Source: CAD feature listing. Evaluate the final solid. Frame: model axes, mm. Give positions to 0.01 mm unless a question says otherwise; leave off trailing zeros. Write each loop counter-clockwise with the first axis right and the second up, starting at its lowest first coordinate (ties: lowest second). Pieces come first, ordered by that corner, then holes. Notation, with made-up numbers: M -7,53 L 22,53 A8 ccw 22,60 Z; hole C -31.5,69 d11. An arc over 180 degrees is marked long. Use CSV: the item, a comma, the result in double quotes. Start each with the question number.
from build123d import *

# Parameters (mm, degrees)
RESSALTO_EXTRUS_O1_DEPTH = 2


with BuildPart() as part:
    # Esboço1 → Ressalto-extrusão1 (new body)
    with BuildSketch(Plane(origin=(0, 0, 0), x_dir=(0, 0, -1), z_dir=(1, 0, 0))):
        with BuildLine():
            Line((0, 0), (-10, 0))
            Line((-10, 0), (-10, 8))
            Line((-10, 8), (-18, 8))
            Line((-18, 8), (-18, 13))
            Line((-18, 13), (-31, 13))
            Line((-31, 13), (-31, 8))
            Line((-31, 8), (-39, 8))
            Line((-39, 8), (-37, 6))
            Line((-37, 6), (-39.121320344, 3.878679656))
            Line((-39.121320344, 3.878679656), (-47.606601718, 12.363961031))
            Line((-47.606601718, 12.363961031), (-60, 12.363961031))
            Line((-60, 12.363961031), (-60.666666667, 10.478342948))
            Line((-60.666666667, 10.478342948), (-63, 11.303300859))
            Line((-63, 11.303300859), (-65.666666667, 3.760828526))
            Line((-65.666666667, 3.760828526), (-63.333333333, 2.935870615))
            Line((-63.333333333, 2.935870615), (-65.303300859, -2.636038969))
            Line((-65.303300859, -2.636038969), (-70, -2.636038969))
            Line((-70, -2.636038969), (-70, 0.363961031))
            Line((-70, 0.363961031), (-77, 0.363961031))
            Line((-77, 0.363961031), (-77, -2.636038969))
            Line((-77, -2.636038969), (-80, -2.636038969))
            Line((-80, -2.636038969), (-78, -9.636038969))
            Line((-78, -9.636038969), (-105.645751311, -9.636038969))
            Line((-105.645751311, -9.636038969), (-106.822875656, -5.813163314))
            Line((-106.822875656, -5.813163314), (-103, -4.636038969))
            Line((-103, -4.636038969), (-104.765686517, 1.098274514))
            Line((-104.765686517, 1.098274514), (-107.645751311, 0.21145666))
            Line((-107.645751311, 0.21145666), (-110, 7.857207972))
            Line((-110, 7.857207972), (-126.395448513, 3.363961031))
            Line((-126.395448513, 3.363961031), (-126.9240658, 5.292837326))
            Line((-126.9240658, 5.292837326), (-135.121790056, 3.046213856))
            ThreePointArc((-135.121790056, 3.046213856), (-136.964910243, 4.096408112), (-135.914715987, 5.939528299))
            Line((-135.914715987, 5.939528299), (-127.71699173, 8.18615177))
            Line((-127.71699173, 8.18615177), (-128.813209852, 12.18615177))
            ThreePointArc((-128.813209852, 12.18615177), (-140.849618713, 9.983199212), (-151.392124565, 3.771620619))
            Line((-151.392124565, 3.771620619), (-149.199688323, -4.228379381))
            Line((-149.199688323, -4.228379381), (-155.950755357, -6.078539886))
            Line((-155.950755357, -6.078539886), (-156, -16.078539886))
            Line((-156, -16.078539886), (-134, -16))
            Line((-134, -16), (-134, -11.101020514))
            ThreePointArc((-134, -11.101020514), (-133, -10.101020514), (-132, -11.101020514))
            Line((-132, -11.101020514), (-132, -16))
            Line((-132, -16), (-120, -16))
            Line((-120, -16), (-118, -14))
            Line((-118, -14), (-39, -14))
            Line((-39, -14), (-29, -16))
            Line((-29, -16), (-29, -11))
            ThreePointArc((-29, -11), (-28, -10), (-27, -11))
            Line((-27, -11), (-27, -16))
            Line((-27, -16), (-7, -13))
            Line((-7, -13), (-7, -8.5))
            ThreePointArc((-7, -8.5), (-5.5, -7), (-4, -8.5))
            Line((-4, -8.5), (-4, -13))
            Line((-4, -13), (0, -10))
            Line((0, -10), (0, 0))
        make_face()
    extrude(amount=RESSALTO_EXTRUS_O1_DEPTH)


solid = part.part
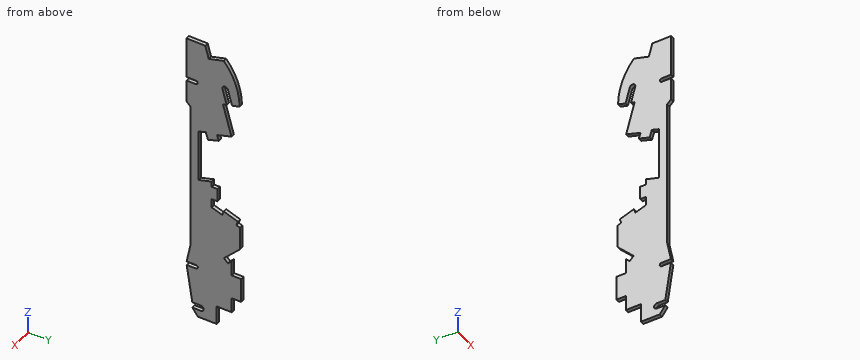
1. Section B-B on z = 81.5. Return loops of the section in (x, y), then the cut area to 3 significant figures.
2. Line query: probe 1 along Z at (x, y) = (1.1, -1.5); probe 2 along Z at (x, y) = (0.1, 9.5); probe 3 along Z at (x, y) = (0.7, -3). Output: solid intervals per line, ascending.
3. Section A-A on z = 5.5. Return loops of the section in (x, y).
4. First-contact query: pin 1 (1 mm diameter, centred on x = 1, y = -0.5, fed in from +Z); pin 2 (0.6 mm diameter, centred on x = 1.5, z = 6, fed in from +Y); pin 3 (0.6 mm diameter, centred on x = 1, y = -12.5, fed in from -Z). Flat tips, straight axial feed; report the tip coordinate or a pass-through.
Resolved:
1,outline,"M 0,-14 L 2,-14 L 2,-9.64 L 0,-9.64 Z"
1,area,"8.73 mm2"
2,probe 1,"z = 0 to 64.9, 70 to 77, 103.97 to 149.95"
2,probe 2,"z = 18 to 31, 44.74 to 63.64, 128.08 to 142.08"
2,probe 3,"z = 0 to 79.9, 103.5 to 149.54"
3,outline,"M 0,-7 L 2,-7 L 2,0 L 0,0 Z"
4,pin 1,"stops at z = 150.36"
4,pin 2,"stops at y = 0"
4,pin 3,"stops at z = 2.93"
